Drawing for the job (mm, zero at the part's lowest x, y, z). A direction names the side the tool comes from. Round coordinates to 2 decimals unless told otherwise and drop trailing zeros. Write each loop counter-clockwise with the first axis right and the second up, starting at its lowest first coordinate (ties: lowest second). Pieces come first, ordered by that corner, then holes.
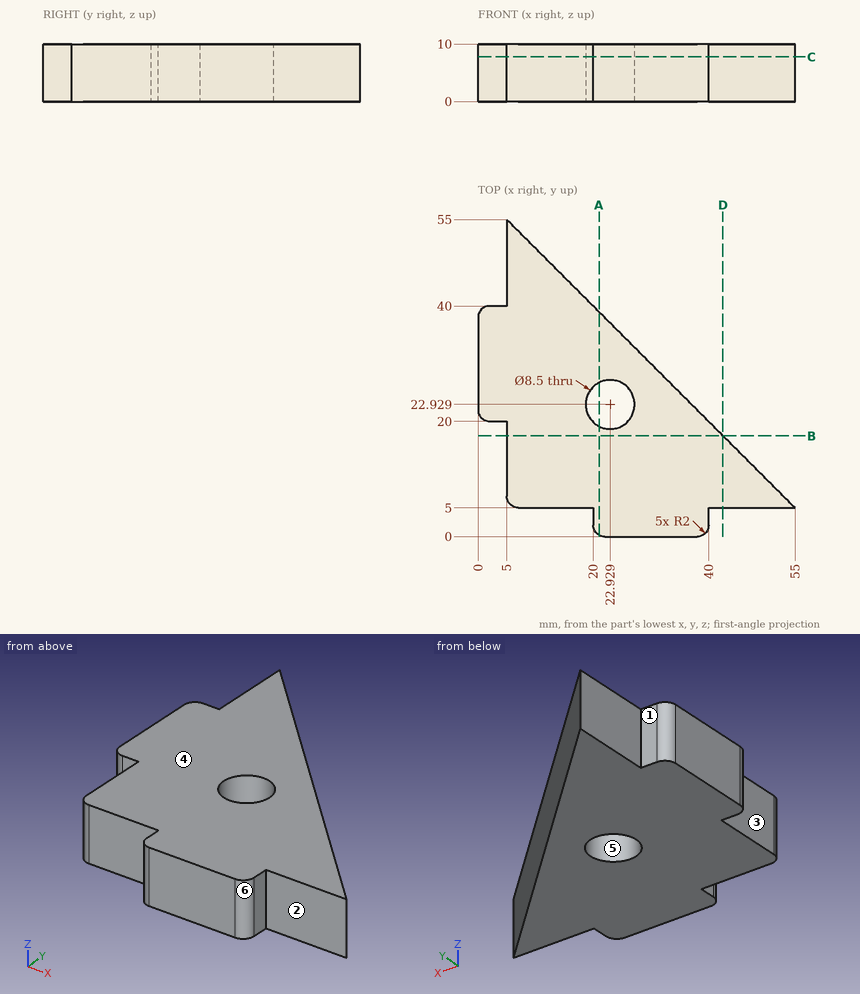
1) Wall check: probe 1 along Y at (x, z) = (25.5, 4.25) (1 decimal); probe 2 along Y at (x, z) = (20.5, 5.25); probe 3 along Y at (x, z) = (2.5, 9.25). Give the ranges that are in metal, low to high.
2) Pull direction X, two halves, no side cores. Call the marked faces 4, 5 and 6: released by +X, released by -X, zero draft, split by the parting line, or undercut.
3) Cut at A-A on x = 21. List the corners of the cut face in (y, z).
4) Flat gauge pins, fed straight in: pin 1 Ø5 at (y, z) = (7, 5.5) entering from -X; pin 2 Ø3.5 at (x, z) = (3.5, 6.5) entering from +Y; pin 3 Ø3.5 at (x, z) = (4, 6) entering from -Y; pin 4 Ø5 at (y, z) = (36, 4.5) entering from -X. Where does each tip first touch, or does it go through?
5) Cut at D-D on x = 42.5. List the corners of the cut face in (y, z).
6) Cut at B-B on y = 17.5. List the corners of the cut face in (x, z).
7) Cut at C-C on z = 7.75. List the corners of the cut face in (x, y).
8) Which spindle directions (+Z, -Z, +X, -X, +Y, -Y) get a long thin tool onto all of the face, cutting with end or side? Do the marked faces 1, 2 and 3. Say none if no direction does.
Result sheet:
1. probe 1: y = 0 to 19.5, 26.3 to 34.5
1. probe 2: y = 0.68 to 19.44, 26.42 to 39.5
1. probe 3: y = 20 to 40
2. face 4: zero draft
2. face 5: undercut
2. face 6: released by +X
3. outline: (0.27, 0) - (19.14, 0) - (19.14, 10) - (0.27, 10) - close; (26.72, 0) - (39, 0) - (39, 10) - (26.72, 10) - close
4. pin 1: stops at x = 5
4. pin 2: stops at y = 55
4. pin 3: stops at y = 5.44
4. pin 4: stops at x = 0
5. outline: (5, 0) - (17.5, 0) - (17.5, 10) - (5, 10) - close
6. outline: (5, 0) - (42.5, 0) - (42.5, 10) - (5, 10) - close
7. outline: (0, 22) arc R2 ccw to (2, 20) - (5, 20) - (5, 7) arc R2 ccw to (7, 5) - (20, 5) - (20, 2) arc R2 ccw to (22, 0) - (38, 0) arc R2 ccw to (40, 2) - (40, 5) - (55, 5) - (5, 55) - (5, 40) - (2, 40) arc R2 ccw to (0, 38) - close; hole circle Ø8.5 at (22.93, 22.93)
8. face 1: +Z, -Z, -X, +Y
8. face 2: +Z, -Z, +X, -Y
8. face 3: +Z, -Z, -X, -Y
